Work out the finished part from the listing and answer in its coordinate system (mm). Give positions to 0.01 mm unless a question says otherwise; leave off trailing zeros. Loops run counter-clockwise (first coordinate to the right, second up) from the corner with the lowest first, then second, coordinate; pieces in that order, holes last. Notation, with made-up numbers: (57, 7) - (84, 7) arc R30 cw to (84, 46) - close; hole circle Ø6 at (-14, -23.75). An arc over 180 degrees is marked (long way). One line per question, with ' | ' between items. Start each with the question number.
1. Find the intervals of material crossed by line 1 (Y direction, x = -2, z = -32); line 2 (X direction, y = 2.75, z = -3); line 3 (Z direction, x = -3.5, y = 4.5), in increasing order.
2. Section A-A (z = -4) is taken. Determine the outline of the cut face in (x, y).
3. Each of these flat-tipped pins is pushed along its axis until it touches: pin 1 (3.5 mm diameter, centred on x = -1.5, y = 2.5, fed in from +Z); pin 2 (3 mm diameter, centred on y = 3.5, z = -31.5, fed in from -X). Where does it stop, or does it pass through?
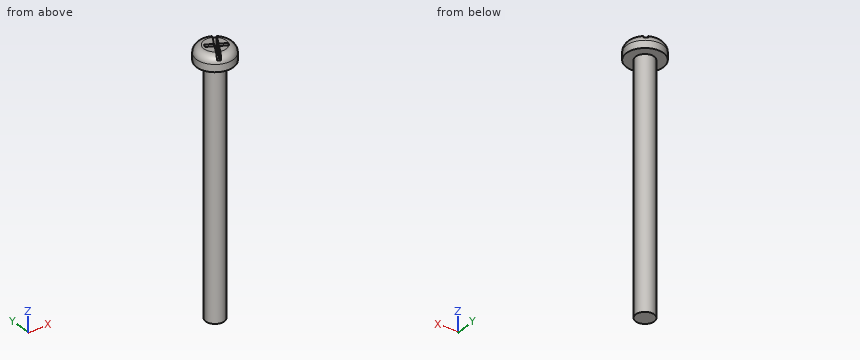
from build123d import *

# Parameters (mm, degrees)
SZKIC1_R                    = 3
DODANIE_WYCI_GNI_CIE2_DEPTH = 2.4
SZKIC2_R                    = 1.5
DODANIE_WYCI_GNI_CIE3_DEPTH = 40
ZAOKR_GLENIE2_R             = 1.2
WYTNIJ_WYCI_GNI_CIE1_DEPTH  = 1.94


with BuildPart() as part:
    # Szkic1 → Dodanie-wyciągnięcie2 (new body)
    with BuildSketch(Plane.XY):
        with Locations((-1.860516246, 2.732142857)):
            Circle(SZKIC1_R)
    extrude(amount=DODANIE_WYCI_GNI_CIE2_DEPTH)

    # Szkic2 → Dodanie-wyciągnięcie3 (add)
    with BuildSketch(Plane(origin=(0, 0, 0), x_dir=(-1, 0, 0), z_dir=(0, 0, -1))):
        with Locations((1.860516246, 2.732142857)):
            Circle(SZKIC2_R)
    extrude(amount=DODANIE_WYCI_GNI_CIE3_DEPTH)

    # Zaokrąglenie2
    zaokr_glenie2_edges = [part.edges().sort_by_distance(p)[0] for p in [
        (-4.860516246, 2.732142857, 2.4),
    ]]
    fillet(zaokr_glenie2_edges, radius=ZAOKR_GLENIE2_R)

    # Szkic3 → Wytnij-wyciągnięcie1 (cut)
    with BuildSketch(Plane.XY.offset(2.4)):
        with BuildLine():
            Line((-1.859548318, 2.959091853), (-0.575649693, 5.316481314))
            ThreePointArc((-0.575649693, 5.316481314), (-0.297886623, 5.158637444), (-0.039271083, 4.97106076))
            Line((-0.039271083, 4.97106076), (-1.329373025, 2.669425378))
            Line((-1.329373025, 2.669425378), (-0.183967515, 2.043621837))
            ThreePointArc((-0.183967515, 2.043621837), (-0.320475658, 1.776553075), (-0.499159616, 1.535654258))
            Line((-0.499159616, 1.535654258), (-1.621312108, 2.148584891))
            Line((-1.621312108, 2.148584891), (-2.819933608, 0.01015725))
            ThreePointArc((-2.819933608, 0.01015725), (-3.083174674, 0.117799023), (-3.33454353, 0.250826496))
            Line((-3.33454353, 0.250826496), (-2.145142944, 2.434706401))
            Line((-2.145142944, 2.434706401), (-3.258687897, 3.042935511))
            ThreePointArc((-3.258687897, 3.042935511), (-3.162842423, 3.328316127), (-3.009463836, 3.587359481))
            Line((-3.009463836, 3.587359481), (-1.859548318, 2.959091853))
        make_face()
    extrude(amount=-WYTNIJ_WYCI_GNI_CIE1_DEPTH, mode=Mode.SUBTRACT)


solid = part.part
Conclusion:
1) line 1: 1.24 to 4.23 | line 2: -3.36 to -0.36 | line 3: 0 to 2.23
2) outline: circle Ø3 at (-1.86, 2.73)
3) pin 1: z = 2.4 | pin 2: x = -3.36
